CAD build for the part. Positions are in the model's coordinates, mm. A direction names the side the tool comes from. Give positions to 0.01 mm unless a question says otherwise; leave off trailing zeros. Write each loop counter-clockwise with the first axis right and the second up, starting at its lowest first coordinate (ties: lowest second). Pieces come first, ordered by that corner, then holes. Notation, with made-up numbers: (-37.5, 53) - (2.5, 53) arc R17 cw to (2.5, 68) - close; hole circle Ø4 at (17, 17). An arc over 180 degrees is marked (long way). Answer as a JSON object with one key per item and string values.
Autodesk Inventor part; units mm, degrees
ref_plane "YZ Plane" through (0, 0, 0) normal (1, 0, 0) x (0, 1, 0)
ref_plane "XZ Plane" through (0, 0, 0) normal (0, 1, 0) x (-1, 0, 0)
ref_plane "XY Plane" through (0, 0, 0) normal (0, 0, 1) x (1, 0, 0)
sketch "Sketch2" plane through (0, 0, 0) normal (0, 1, 0) x (-1, 0, 0)
  line L0 (25, -25) -> (-25, -25)
  line L1 (-25, -25) -> (-25, 25)
  line L2 (-25, 25) -> (25, 25)
  line L3 (25, 25) -> (25, -25)
  line L4 (25, -25) -> (-25, 25) construction
  line L5 (-25, -25) -> (25, 25) construction
  line L6 (35, 35) -> (-35, 35)
  line L7 (-35, 35) -> (-35, -35)
  line L8 (-35, -35) -> (35, -35)
  line L9 (35, -35) -> (35, 35)
  point P0 (0, 0)
  dimension "d0" = 50
  dimension "d1" = 10
  dimension "d19" = 50
extrude "Extrusion1" add sketch "Sketch2" along normal mid plane 30
sketch "Sketch3" plane through (0, -15, 0) normal (0, -1, 0) x (1, 0, 0)
  line L0 (35, -35) -> (35, 35)
  line L1 (35, 35) -> (-35, 35)
  line L2 (-35, 35) -> (-35, -35)
  line L3 (-35, -35) -> (35, -35)
  point P0 (0, 0)
extrude "Extrusion2" add sketch "Sketch3" against normal blind 10
chamfer "Chamfer1" distance 10 angle 45 16 edges at (35, 0, 35) (25, 5, 25) (-25, 5, 25) (-35, 0, 35) (-25, 5, -25) (25, 5, -25) (-35, 0, -35) (35, 0, -35) (0, -5, -25) (25, -5, 0) (0, -5, 25) (-25, -5, 0) (0, -15, -35) (35, -15, 0) (0, -15, 35) (-35, -15, 0)
sketch "Sketch4" plane through (35, -5, -25) normal (1, 0, 0) x (0, 0, -1)
  line L0 (0, 20) -> (0, 0) construction
  line L1 (-50, 20) -> (0, 20) construction
  line L2 (-16.3397, 30) -> (-16.3397, 20)
  line L3 (-16.3397, 20) -> (-25, 15)
  line L4 (-25, 15) -> (-33.6603, 20)
  line L5 (-33.6603, 20) -> (-33.6603, 30)
  line L6 (-33.6603, 30) -> (-25, 35)
  line L7 (-25, 35) -> (-16.3397, 30)
  point P0 (-25, 5)
  point P1 (-25, 25)
  dimension "d9" = 10
  dimension "d10" = 5
  dimension "d20" = 0
extrude "Extrusion3" cut sketch "Sketch4" against normal blind 10
sketch "Sketch5" plane through (0, 15, 0) normal (0, 1, 0) x (1, 0, 0)
  line L0 (-25, 25) -> (-25, 35) construction
  circle A0 centre (-25, 25) radius 2.5
  line L1 (25, 25) -> (35, 25) construction
  circle A1 centre (25, 25) radius 2.5
  line L2 (-25, -25) -> (-35, -25) construction
  circle A2 centre (-25, -25) radius 2.5
  line L3 (-25, -25) -> (25, -25) construction
  circle A3 centre (25, -25) radius 2.5
  point P0 (0, 0)
  dimension "d13" = 5
  dimension "d14" = 5
  dimension "d15" = 5
  dimension "d16" = 5
extrude "Extrusion4" cut sketch "Sketch5" against normal blind 10
sketch "Sketch6" plane through (-35, -5, -25) normal (-1, 0, 0) x (0, 0, 1)
  line L0 (0, 20) -> (50, 20) construction
  line L1 (9.5, 14.9) -> (40.5, 14.9)
  line L2 (40.5, 14.9) -> (40.5, 20)
  line L3 (40.5, 20) -> (9.5, 20)
  line L4 (9.5, 20) -> (9.5, 14.9)
  point P0 (25, 5)
  point P1 (25, 20)
  dimension "d21" = 31
  dimension "d22" = 5.1
extrude "Extrusion5" cut sketch "Sketch6" against normal blind 12
sketch "Sketch7" plane through (-35, 9.9, 15.5) normal (0, 1, 0) x (1, 0, 0)
  line L0 (0, 0) -> (10.5, 0) construction
  line L1 (0, 31) -> (10.5, 31) construction
  circle A0 centre (5, 21) radius 2.5
  circle A1 centre (5, 10) radius 2.5
  point P0 (10, 0)
  point P1 (10, 31)
  point P2 (35, 15.5)
  dimension "d25" = 5
  dimension "d26" = 5
  dimension "d27" = 10
  dimension "d28" = 10
extrude "Extrusion6" cut sketch "Sketch7" against normal blind 10
chamfer "Chamfer2" distance 1 angle 45 6 edges at (-32.5, 9.9, 5.5) (-32.5, 9.9, -5.5) (-27.5, 15, -25) (-27.5, 15, 25) (22.5, 15, 25) (22.5, 15, -25)
properties part number "pokemon_ball_white"
(1) Saw through at C-C, the plane x = -8.5. Give the cut face in (y, z).
Answer key:
{"outline": "(-15, -25) - (-5, -35) - (15, -35) - (15, -25) - (5, -25) - (-5, -15) - (-5, 15) - (5, 25) - (15, 25) - (15, 35) - (-5, 35) - (-15, 25) - close"}
(2) Saw through at B-B, the plane z = 16.5. Give the cut face in (x, y).
Answer key:
{"outline": "(-35, -5) - (-25, -15) - (25, -15) - (35, -5) - (35, 15) - (23.5, 15) - (23.5, 5) - (15, -3.5) - (-15, -3.5) - (-23.5, 5) - (-23.5, 15) - (-35, 15) - close"}
(3) Flat gauge pins, fed straight in: P1, Ø8, axis at x = -24.5, z = -5, coming from the +Y side; P2, Ø1.5, axis at x = -29, y = 12.5, coming from the -Z side; P3, Ø2.5, axis at x = 25.5, z = 25, coming from the +Y side. Where does each tip first touch, or does it go through?
Answer key:
{"P1": "stops at y = 9.9", "P2": "stops at z = -31.75", "P3": "stops at y = 5"}
(4) Saw through at D-D, the plane y = 6. Give the cut face in (x, z).
Answer key:
{"outline": "(-35, -25) - (-25, -35) - (25, -35) - (35, -25) - (35, 25) - (25, 35) - (-25, 35) - (-35, 25) - close; hole circle Ø5 at (-30, -5.5); hole circle Ø5 at (-30, 5.5); hole circle Ø5 at (-25, -25); hole circle Ø5 at (-25, 25); hole (-25, -15) - (-15, -25) - (15, -25) - (25, -15) - (25, 15) - (15, 25) - (-15, 25) - (-25, 15) - close; hole circle Ø5 at (25, -25); hole circle Ø5 at (25, 25)"}
(5) Probe L1, parallel to Z at x = -25, y = 10.5; L2, parallel to Z at x = -30, y = 4; L3, parallel to Z at x = -1, y = 9.5. List the from-to ranges inside material, lowest first. Write a range as [from, to].
Answer key:
{"L1": "z = [-35, -27.5], [-22.5, -15.5], [15.5, 22.5], [27.5, 35]", "L2": "z = [-30, -8], [-3, 3], [8, 30]", "L3": "z = [-35, -25], [25, 35]"}
(6) Pull direction Z, two halves, no side cores. Call faces 1 (the face through (-30, 5, -30)), 2 (the face through (0, 0, 20)), 3 (the face through (35, 5, 0)): pulls with the +Z half, pulls with the -Z half, needs draft (parallel to the pull), parting line crosses it, or undercut.
Answer key:
{"face 1": "pulls with the -Z half", "face 2": "undercut", "face 3": "needs draft"}
(7) Saw through at A-A, the plane y = -3. Give the cut face in (x, z).
Answer key:
{"outline": "(-35, -25) - (-25, -35) - (25, -35) - (35, -25) - (35, 25) - (25, 35) - (-25, 35) - (-35, 25) - close; hole (-17, -15) - (-15, -17) - (15, -17) - (17, -15) - (17, 15) - (15, 17) - (-15, 17) - (-17, 15) - close"}
(8) 3-axis set-ups, long thin cutter, end or side, ignore diameter. For faces 4 (the face through (30, -10, 0)), 5 (the face through (0, -5, 0)): which of +Z, -Z, +X, -X, +Y, -Y reach the whole face in a straight line?
Answer key:
{"face 4": "+Z, -Z, +X, -Y", "face 5": "+Y"}
